Geometry check sheet. Reference: the model listing, model coordinates, mm. A direction names the side the tool comes from. Give positions to 0.01 mm unless a question says otherwise; leave off trailing zeros. Write each loop counter-clockwise with the first axis right and the second up, starting at its lowest first coordinate (ties: lowest second). Pieces come first, ordered by that corner, then holes.
(1) Mould release check, pull along Z, two halves, no side actions. Record for faces 1 (the flat face through (-2, 0.5, 0)), 2 (the flat face through (-3.808, 6.409, 3.828)), 3 (the flat face through (0, 6, -5.399)), 4 (the flat face through (-3.7, 13, -3.7)): +Z half, -Z half, draft (parallel to the pull), parting line (faces both ways), or undercut.
(2) Tool access check on faces 5 (the flat face through (-3.7, 13, 3.7)), 6 (the cylindrical face through (-4.614, 6.409, 1.926)), 7 (the cylindrical face through (4.625, 6.409, 1.901)). Record the directions out of +Z, -Z, +X, -X, +Y, -Y that give a thin tool (end or side, any length) a straight path to the whole face; none if there is none.
(3) Depth check by flat-ended pin: P1, Ø1, axis at y = 10, z = -3, coming from the -X side; P2, Ø5, axis at x = 4, y = 7.5, coming from the +Z side; P3, Ø0.9, axis at x = 4, z = 4, coming from the +Y side. Enter the tip coordinate at first touch or a pass-through.
(4) Thickness scan on line 1 along Z through (x, y) = (0, 9.5); line 2 along X through (y, z) = (7.25, 0); line 3 along X through (y, z) = (3.25, 5). Record the ranges inside material, lowest first.
(5) Cross-section at C-C (z = 0). Record the boundary of the cut face in (x, y), and give its area (3 significant figures).
(6) Cross-section at B-B (x = 0). Record the boundary of the cut face in (y, z), and give its area (3 significant figures).
Autodesk Inventor part; units mm, degrees
ref_plane "YZ Plane" through (0, 0, 0) normal (1, 0, 0) x (0, 1, 0)
ref_plane "XY Plane" through (0, 0, 0) normal (0, 0, 1) x (1, 0, 0)
sketch "Sketch1" plane through (0, 0, 0) normal (0, 1, 0) x (-1, 0, 0)
  arc A0 (1.5, 2.5981) -> (1.5, -2.5981) centre (0, 0) ccw
  line L0 (1.5, 2.5981) -> (1.5, -2.5981)
  line L1 (1.5, 0) -> (-3, 0) construction
  circle A1 centre (0, 0) radius 5
  dimension "d0" = 6
  dimension "d1" = 4.5
  dimension "d2" = 10
extrude "Extrusion1" add sketch "Sketch1" along normal blind 12
sketch "Sketch2" plane through (0, 12, 0) normal (0, 1, 0) x (1, 0, 0)
  circle A0 centre (0, 0) radius 5
extrude "Extrusion2" add sketch "Sketch2" along normal blind 2
chamfer "Chamfer1" distance 1 angle 45 1 edges at (-5, 14, 0)
sketch "Sketch3" plane through (0, 0, 0) normal (0, 1, 0) x (-1, 0, 0)
  circle A0 centre (0, 0) radius 5
  line L0 (4.899, 1) -> (5.399, 1)
  line L1 (5.399, 1) -> (5.399, -1)
  line L2 (5.399, -1) -> (4.899, -1)
  arc A1 (4.899, -1) -> (4.899, 1) centre (0, 0) ccw
  dimension "d10" = 2
  dimension "d11" = 0.5
  dimension "d12" = 1
extrude "Extrusion3" add sketch "Sketch3" along normal blind 13 contours A0 L0 L1 L2
pattern_circular "Circular Pattern1" count 8 over 360 about axis through (0, 0, 0) along (0, 1, 0) of "Extrusion3"
chamfer "Chamfer2" distance 1 angle 45 2 edges at (-1.5, 0, 0) (3, 0, 0)
properties part number "Pot-knob"
Reply:
1. face 1: undercut
1. face 2: +Z half
1. face 3: -Z half
1. face 4: draft
2. face 5: +Z, -X, +Y
2. face 6: -X, +Y, -Y
2. face 7: +X, +Y, -Y
3. P1: stops at x = -4.52
3. P2: stops at z = 4.77
3. P3: stops at y = 13
4. line 1: z = -5.4 to -3, 3 to 5.4
4. line 2: x = -5.4 to -1.5, 3 to 5.4
4. line 3: x = -1 to 1
5. outline: (-5.4, 0) - (-2.5, 0) - (-1.5, 1) - (-1.5, 12) - (3, 12) - (3, 1) - (4, 0) - (5.4, 0) - (5.4, 13) - (5, 13) - (4, 14) - (-4, 14) - (-5, 13) - (-5.4, 13) - close
5. area: 94.4 mm2
6. outline: (0, -5.4) - (13, -5.4) - (13, -5) - (14, -4) - (14, 4) - (13, 5) - (13, 5.4) - (0, 5.4) - (0, 4) - (1, 3) - (12, 3) - (12, -3) - (1, -3) - (0, -4) - close
6. area: 76.4 mm2
